Autodesk Inventor part; units mm, degrees
ref_plane "YZ Plane" through (0, 0, 0) normal (1, 0, 0) x (0, 1, 0)
ref_plane "XZ Plane" through (0, 0, 0) normal (0, 1, 0) x (-1, 0, 0)
ref_plane "XY Plane" through (0, 0, 0) normal (0, 0, 1) x (1, 0, 0)
sketch "Szkic1" plane through (0, 0, 0) normal (1, 0, 0) x (0, 1, 0)
  line L0 (-37, 37) -> (37, 37)
  line L1 (37, 37) -> (37, -37)
  line L2 (37, -37) -> (-37, -37)
  line L3 (-37, -37) -> (-37, 37)
  line L4 (-37, 37) -> (37, -37) construction
  line L5 (37, 37) -> (-37, -37) construction
  point P0 (0, 0)
  dimension "d0" = 74
  dimension "d1" = 74
extrude "Wyciągnięcie proste1" add sketch "Szkic1" along normal blind 18
sketch "Szkic2" plane through (18, 0, 0) normal (1, 0, 0) x (0, 0, -1)
  circle A0 centre (-27.4, 31) radius 2.85
  line L0 (37, 37) -> (-37, 37)
  line L1 (-37, 37) -> (-37, -37)
  circle A1 centre (-27.4, 0) radius 2.85
  circle A2 centre (-27.4, -31) radius 2.85
  circle A3 centre (27.4, 31) radius 2.85
  line L2 (37, -37) -> (37, 37)
  circle A4 centre (27.4, 0) radius 2.85
  circle A5 centre (27.4, -31) radius 2.85
  line L3 (-29.8537, 35.25) -> (-24.9463, 35.25)
  line L4 (-24.9463, 35.25) -> (-22.4925, 31)
  line L5 (-22.4925, 31) -> (-24.9463, 26.75)
  line L6 (-24.9463, 26.75) -> (-29.8537, 26.75)
  line L7 (-29.8537, 26.75) -> (-32.3075, 31)
  line L8 (-32.3075, 31) -> (-29.8537, 35.25)
  line L9 (-29.8537, 4.25) -> (-24.9463, 4.25)
  line L10 (-24.9463, 4.25) -> (-22.4925, 0)
  line L11 (-22.4925, 0) -> (-24.9463, -4.25)
  line L12 (-24.9463, -4.25) -> (-29.8537, -4.25)
  line L13 (-29.8537, -4.25) -> (-32.3075, 0)
  line L14 (-32.3075, 0) -> (-29.8537, 4.25)
  line L15 (-29.8537, -26.75) -> (-24.9463, -26.75)
  line L16 (-24.9463, -26.75) -> (-22.4925, -31)
  line L17 (-22.4925, -31) -> (-24.9463, -35.25)
  line L18 (-24.9463, -35.25) -> (-29.8537, -35.25)
  line L19 (-29.8537, -35.25) -> (-32.3075, -31)
  line L20 (-32.3075, -31) -> (-29.8537, -26.75)
  line L21 (29.8537, 35.25) -> (32.3075, 31)
  line L22 (32.3075, 31) -> (29.8537, 26.75)
  line L23 (29.8537, 26.75) -> (24.9463, 26.75)
  line L24 (24.9463, 26.75) -> (22.4925, 31)
  line L25 (22.4925, 31) -> (24.9463, 35.25)
  line L26 (24.9463, 35.25) -> (29.8537, 35.25)
  line L27 (29.8537, 4.25) -> (32.3075, 0)
  line L28 (32.3075, 0) -> (29.8537, -4.25)
  line L29 (29.8537, -4.25) -> (24.9463, -4.25)
  line L30 (24.9463, -4.25) -> (22.4925, 0)
  line L31 (22.4925, 0) -> (24.9463, 4.25)
  line L32 (24.9463, 4.25) -> (29.8537, 4.25)
  line L33 (29.8537, -26.75) -> (32.3075, -31)
  line L34 (32.3075, -31) -> (29.8537, -35.25)
  line L35 (29.8537, -35.25) -> (24.9463, -35.25)
  line L36 (24.9463, -35.25) -> (22.4925, -31)
  line L37 (22.4925, -31) -> (24.9463, -26.75)
  line L38 (24.9463, -26.75) -> (29.8537, -26.75)
  point P0 (0, 0)
  point P1 (27.4, -26.75)
  dimension "d4" = 6
  dimension "d5" = 5.7
  dimension "d6" = 9.6
  dimension "d7" = 31
  dimension "d8" = 31
  dimension "d9" = 5.7
  dimension "d10" = 5.7
  dimension "d11" = 9.6
  dimension "d12" = 5.7
  dimension "d13" = 5.7
  dimension "d14" = 5.7
  dimension "d15" = 8.5
  dimension "d16" = 8.5
  dimension "d17" = 8.5
  dimension "d18" = 8.5
  dimension "d19" = 8.5
  dimension "d20" = 8.5
extrude "Wyciągnięcie proste2" cut sketch "Szkic2" against normal through all contours A0 | A1 | A2 | A3 | A4 | A5
extrude "Wyciągnięcie proste3" cut sketch "Szkic2" against normal blind 5 contours A0 | A1 | A2 | A3 | A4 | A5 | L3 L4 L5 L6 L7 L8 | L9 L10 L11 L12 L13 L14 | L15 L16 L17 L18 L19 L20 | L21 L22 L23 L24 L25 L26 | L27 L28 L29 L30 L31 L32 | L33 L34 L35 L36 L37 L38
sketch "Szkic3" plane through (0, -37, 37) normal (0, 0, 1) x (1, 0, 0)
  line L0 (0, 0) -> (0, 74)
  line L1 (0, 72.5) -> (2, 72.5)
  line L2 (2, 72.5) -> (2, 63.5)
  line L3 (2, 63.5) -> (0, 63.5)
  line L4 (0, 63.5) -> (0, 72.5)
  line L5 (0, 74) -> (18, 74)
  line L6 (0, 10.5) -> (2, 10.5)
  line L7 (2, 10.5) -> (2, 1.5)
  line L8 (2, 1.5) -> (0, 1.5)
  line L9 (0, 1.5) -> (0, 10.5)
  point P0 (0, 37)
  point P1 (0, 1.5)
  point P2 (0, 63.5)
  dimension "d25" = 1.5
  dimension "d26" = 9
  dimension "d27" = 2
  dimension "d28" = 2
  dimension "d29" = 9
  dimension "d30" = 1.5
extrude "Wyciągnięcie proste4" cut sketch "Szkic3" against normal through all
sketch "Szkic4" plane through (0, -37, 37) normal (0, 0, 1) x (1, 0, 0)
  line L0 (10.5, 60.5) -> (10.5, 44.5)
  line L1 (10.5, 44.5) -> (16.3, 44.5)
  line L2 (16.3, 44.5) -> (16.3, 50.5)
  line L3 (16.3, 60.5) -> (10.5, 60.5)
  line L4 (16.3, 50.5) -> (18, 50.5)
  line L5 (18, 50.5) -> (18, 54.5)
  line L6 (18, 54.5) -> (16.3, 54.5)
  line L7 (16.3, 54.5) -> (16.3, 60.5)
  line L8 (16.3, 50.5) -> (16.3, 54.5) construction
  line L9 (18, 74) -> (18, 0)
  line L10 (18, 63.75) -> (13, 63.75)
  line L11 (18, 63.75) -> (13, 63.75)
  point P0 (0, 37)
  dimension "d33" = 5.8
  dimension "d34" = 4
  dimension "d35" = 1.7
  dimension "d36" = 6
  dimension "d37" = 16
  dimension "d38" = 3.25
extrude "Wyciągnięcie proste5" cut sketch "Szkic4" against normal blind 20
properties part number "XItemEndCoverConnector" material "Tworzywo sztuczne ABS"
CAD build for the part. Positions are in the model's coordinates, mm. A direction names the side the tool comes from. Give positions to 0.01 mm unless a question says otherwise; leave off trailing zeros. Loops run counter-clockwise (first coordinate to the right, second up) from the corner with the lowest first, then second, coordinate; pieces in that order, holes last. Notation, with made-up numbers: M -2.75,20.5 L 18.25,20.5 A17 cw 18.25,52.5 Z; hole C 47,-16.5 d4. An arc over 180 degrees is marked long. One line per question, with ' | ' between items. Start each with the question number.
1. Saw through at D-D on z = -27.4. State how many separate pieces and enclosed holes the cut face has, plus the area to 3 significant figures.
2. Saw through at B-B on y = 1. Give the cut face in (x, z).
3. Flat gauge pins, fed straight in: pin 1 (1.5 mm diameter, centred on x = 13.5, y = 10.5, fed in from +Z); pin 2 (4.5 mm diameter, centred on y = 29, z = -14.5, fed in from -X). Where does each tip first touch, or does it go through?
4. Two-plate mould, pull along X, no slides. Class faces 6 (the face through (1, -26.5, 1)), 7 (the face through (13, 33, 25)), 8 (the face through (16.3, 20, 27)): pulls with the +X half, pulls with the -X half, needs draft (parallel to the pull), parting line crosses it, or undercut.
5. Saw through at C-C on z = -5.5. Give the cut face in (x, y).
6. Saw through at A-A on x = 5. Give the cut face in (y, z), plus the area to 3 significant figures.
7. 3-axis set-ups, long thin cutter, end or side, ignore diameter. For faces 1 (the face through (2, -31, 1)), 2 (the face through (13, -29, 25)), 3 (the face through (13, 23.5, 27)), 4 (the face through (6.591, 0.125, 30.247)), 5 (the face through (9, -37, -1)): which of +Z, -Z, +X, -X, +Y, -Y reach the whole face in a straight line?
8. Probe L1, parallel to Y at x = 9.5, z = -27.4; L2, parallel to Y at x = 4.5, z = -28.5; L3, parallel to Z at x = 9, y = -2. List the from-to ranges inside material, lowest first. Write a range as from..to.
Result sheet:
1) separate pieces: 4 | enclosed holes: 0 | area: 969 mm^2
2) outline: M 0,-37 L 18,-37 L 18,-31.73 L 13,-31.73 L 13,-30.07 L 0,-30.07 Z; M 0,-24.73 L 13,-24.73 L 13,-23.07 L 18,-23.07 L 18,23.07 L 13,23.07 L 13,24.73 L 0,24.73 Z; M 0,30.07 L 13,30.07 L 13,31.73 L 18,31.73 L 18,37 L 0,37 Z
3) pin 1: stops at z = 17 | pin 2: stops at x = 2
4) face 6: needs draft | face 7: pulls with the +X half | face 8: undercut
5) outline: M 0,-37 L 18,-37 L 18,37 L 0,37 L 0,35.5 L 2,35.5 L 2,26.5 L 0,26.5 L 0,-26.5 L 2,-26.5 L 2,-35.5 L 0,-35.5 Z
6) outline: M -37,-37 L 37,-37 L 37,37 L -37,37 Z; hole C -31,-27.4 d5.7; hole C -31,27.4 d5.7; hole C 0,-27.4 d5.7; hole C 0,27.4 d5.7; hole C 31,-27.4 d5.7; hole C 31,27.4 d5.7 | area: 5,320 mm^2
7) face 1: +Z, -Z, -X | face 2: +X | face 3: +Z | face 4: +X, -X | face 5: +Z, -Z, +X, -X, -Y
8) L1: y = -37..-33.85, -28.15..-2.85, 2.85..28.15, 33.85..37 | L2: y = -37..-33.63, -28.37..-2.63, 2.63..28.37, 33.63..37 | L3: z = -37..-29.43, -25.37..25.37, 29.43..37
